Design review of the part built by this model. Coordinates are the model's own, in mm. Face numbers are marked on the shaded views. A direction names the side the tool comes from. Coordinates: 2 decimals unless noted, no trailing zeros. Write each loop counter-clockwise with the first axis right and the second up, starting at its lowest first coordinate (ties: lowest second). Pieces come first, ordered by that corner, then holes. Notation, with made-up numbers: (10.5, 27.25) - (66.5, 27.25) arc R14 ccw to (66.5, 46.25) - close; hole circle Ø5 at (-16.5, -18.5). An arc over 180 degrees is marked (long way). Answer as a JSON object with one key per item and string values.
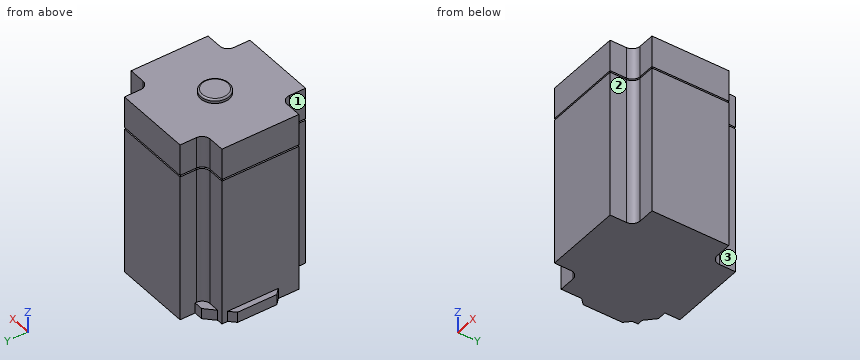
```python
from build123d import *

# Parameters (mm, degrees)
Y_KSEKLIK_EKSTR_ZYON1_DEPTH     = 13
Y_KSEKLIK_EKSTR_ZYON2_DEPTH     = 224
KES_EKSTR_ZYON1_DEPTH           = 1
KES_EKSTR_ZYON1_TAPER           = 45
KES_EKSTR_ZYON1_OTHER_WAY_DEPTH = 1
KES_EKSTR_ZYON1_OTHER_WAY_TAPER = 45
IZIM8_R                         = 17.581787387
Y_KSEKLIK_EKSTR_ZYON3_DEPTH     = 5
RADYUS2_R                       = 2


with BuildPart() as part:
    # Çizim1 → Yükseklik-Ekstrüzyon1 (new body)
    with BuildSketch(Plane.XY):
        Polygon((-58.626768768, 58.968306861), (-84.598484816, 33.394607486), (-84.598484816, -15.059977091), (-58.626768768, -41.031693139), (-10.172184191, -41.031693139), (15.401515184, -15.059977091), (15.401515184, 32.642615461), (-10.924176216, 58.968306861), align=None)
    extrude(amount=Y_KSEKLIK_EKSTR_ZYON1_DEPTH)

    # Çizim2 → Yükseklik-Ekstrüzyon2 (add)
    with BuildSketch(Plane.XY):
        with BuildLine():
            Line((47.5, 57.5), (47.5, 77.5))
            Line((47.5, 77.5), (-47.5, 77.5))
            Line((-47.5, 77.5), (-47.5, 57.5))
            ThreePointArc((-47.5, 57.5), (-50.428932188, 50.428932188), (-57.5, 47.5))
            Line((-57.5, 47.5), (-77.5, 47.5))
            Line((-77.5, 47.5), (-77.5, -47.5))
            Line((-77.5, -47.5), (-57.5, -47.5))
            ThreePointArc((-57.5, -47.5), (-50.428932188, -50.428932188), (-47.5, -57.5))
            Line((-47.5, -57.5), (-47.5, -77.5))
            Line((-47.5, -77.5), (47.5, -77.5))
            Line((47.5, -77.5), (47.5, -57.5))
            ThreePointArc((47.5, -57.5), (50.428932188, -50.428932188), (57.5, -47.5))
            Line((57.5, -47.5), (77.5, -47.5))
            Line((77.5, -47.5), (77.5, 47.5))
            Line((77.5, 47.5), (57.5, 47.5))
            ThreePointArc((57.5, 47.5), (50.428932188, 50.428932188), (47.5, 57.5))
        make_face()
    extrude(amount=Y_KSEKLIK_EKSTR_ZYON2_DEPTH)

    # Çizim7 → Kes-Ekstrüzyon1 (cut)
    with BuildSketch(Plane.XY.offset(184)):
        with BuildLine():
            Line((57.5, -56.5), (86.5, -56.5))
            Line((86.5, -56.5), (86.5, 56.5))
            Line((86.5, 56.5), (57.5, 56.5))
            ThreePointArc((57.5, 56.5), (56.792893219, 56.792893219), (56.5, 57.5))
            Line((56.5, 57.5), (56.5, 86.5))
            Line((56.5, 86.5), (-56.5, 86.5))
            Line((-56.5, 86.5), (-56.5, 57.5))
            ThreePointArc((-56.5, 57.5), (-56.792893219, 56.792893219), (-57.5, 56.5))
            Line((-57.5, 56.5), (-86.5, 56.5))
            Line((-86.5, 56.5), (-86.5, -56.5))
            Line((-86.5, -56.5), (-57.5, -56.5))
            ThreePointArc((-57.5, -56.5), (-56.792893219, -56.792893219), (-56.5, -57.5))
            Line((-56.5, -57.5), (-56.5, -86.5))
            Line((-56.5, -86.5), (56.5, -86.5))
            Line((56.5, -86.5), (56.5, -57.5))
            ThreePointArc((56.5, -57.5), (56.792893219, -56.792893219), (57.5, -56.5))
        make_face()
        with BuildLine():
            Line((-46.5, -76.5), (46.5, -76.5))
            Line((46.5, -76.5), (46.5, -57.5))
            ThreePointArc((46.5, -57.5), (49.721825407, -49.721825407), (57.5, -46.5))
            Line((57.5, -46.5), (76.5, -46.5))
            Line((76.5, -46.5), (76.5, 46.5))
            Line((76.5, 46.5), (57.5, 46.5))
            ThreePointArc((57.5, 46.5), (49.721825407, 49.721825407), (46.5, 57.5))
            Line((46.5, 57.5), (46.5, 76.5))
            Line((46.5, 76.5), (-46.5, 76.5))
            Line((-46.5, 76.5), (-46.5, 57.5))
            ThreePointArc((-46.5, 57.5), (-49.721825407, 49.721825407), (-57.5, 46.5))
            Line((-57.5, 46.5), (-76.5, 46.5))
            Line((-76.5, 46.5), (-76.5, -46.5))
            Line((-76.5, -46.5), (-57.5, -46.5))
            ThreePointArc((-57.5, -46.5), (-49.721825407, -49.721825407), (-46.5, -57.5))
            Line((-46.5, -57.5), (-46.5, -76.5))
        make_face(mode=Mode.SUBTRACT)
    extrude(amount=-KES_EKSTR_ZYON1_DEPTH, taper=KES_EKSTR_ZYON1_TAPER, mode=Mode.SUBTRACT)

    # Çizim7 → Kes-Ekstrüzyon1 other way (cut)
    with BuildSketch(Plane.XY.offset(184)):
        with BuildLine():
            Line((57.5, -56.5), (86.5, -56.5))
            Line((86.5, -56.5), (86.5, 56.5))
            Line((86.5, 56.5), (57.5, 56.5))
            ThreePointArc((57.5, 56.5), (56.792893219, 56.792893219), (56.5, 57.5))
            Line((56.5, 57.5), (56.5, 86.5))
            Line((56.5, 86.5), (-56.5, 86.5))
            Line((-56.5, 86.5), (-56.5, 57.5))
            ThreePointArc((-56.5, 57.5), (-56.792893219, 56.792893219), (-57.5, 56.5))
            Line((-57.5, 56.5), (-86.5, 56.5))
            Line((-86.5, 56.5), (-86.5, -56.5))
            Line((-86.5, -56.5), (-57.5, -56.5))
            ThreePointArc((-57.5, -56.5), (-56.792893219, -56.792893219), (-56.5, -57.5))
            Line((-56.5, -57.5), (-56.5, -86.5))
            Line((-56.5, -86.5), (56.5, -86.5))
            Line((56.5, -86.5), (56.5, -57.5))
            ThreePointArc((56.5, -57.5), (56.792893219, -56.792893219), (57.5, -56.5))
        make_face()
        with BuildLine():
            Line((-46.5, -76.5), (46.5, -76.5))
            Line((46.5, -76.5), (46.5, -57.5))
            ThreePointArc((46.5, -57.5), (49.721825407, -49.721825407), (57.5, -46.5))
            Line((57.5, -46.5), (76.5, -46.5))
            Line((76.5, -46.5), (76.5, 46.5))
            Line((76.5, 46.5), (57.5, 46.5))
            ThreePointArc((57.5, 46.5), (49.721825407, 49.721825407), (46.5, 57.5))
            Line((46.5, 57.5), (46.5, 76.5))
            Line((46.5, 76.5), (-46.5, 76.5))
            Line((-46.5, 76.5), (-46.5, 57.5))
            ThreePointArc((-46.5, 57.5), (-49.721825407, 49.721825407), (-57.5, 46.5))
            Line((-57.5, 46.5), (-76.5, 46.5))
            Line((-76.5, 46.5), (-76.5, -46.5))
            Line((-76.5, -46.5), (-57.5, -46.5))
            ThreePointArc((-57.5, -46.5), (-49.721825407, -49.721825407), (-46.5, -57.5))
            Line((-46.5, -57.5), (-46.5, -76.5))
        make_face(mode=Mode.SUBTRACT)
    extrude(amount=KES_EKSTR_ZYON1_OTHER_WAY_DEPTH, taper=KES_EKSTR_ZYON1_OTHER_WAY_TAPER, mode=Mode.SUBTRACT)

    # Çizim8 → Yükseklik-Ekstrüzyon3 (add)
    with BuildSketch(Plane.XY.offset(224)):
        Circle(IZIM8_R)
    extrude(amount=Y_KSEKLIK_EKSTR_ZYON3_DEPTH)

    # Radyus2
    radyus2_edges = [part.edges().sort_by_distance(p)[0] for p in [
        (-17.581787387, 0, 229),
    ]]
    fillet(radyus2_edges, radius=RADYUS2_R)


solid = part.part
```
(1) To check wall thickness, follow line 1 (Y direction, x = -61, z = 19); line 2 (X direction, y = -11, z = 52.5). State the ranges of each line that lie inside material, in increasing order. Write a range as from..to.
Solved:
{"line 1": "y = -47.5..47.5", "line 2": "x = -77.5..77.5"}
(2) Take a section at A-A, the plane z = 95.5. Write out the cut boundary in (x, y).
Solved:
{"outline": "(-77.5, -47.5) - (-57.5, -47.5) arc R10 cw to (-47.5, -57.5) - (-47.5, -77.5) - (47.5, -77.5) - (47.5, -57.5) arc R10 cw to (57.5, -47.5) - (77.5, -47.5) - (77.5, 47.5) - (57.5, 47.5) arc R10 cw to (47.5, 57.5) - (47.5, 77.5) - (-47.5, 77.5) - (-47.5, 57.5) arc R10 cw to (-57.5, 47.5) - (-77.5, 47.5) - close"}
(3) For pin 1 (6 mm diameter, centred on x = -63, z = 204.5, fed in from -Y); pin 2 (22 mm diameter, centred on x = 67.5, z = 82.5, fed in from +Y); pin 3 (6 mm diameter, centred on y = 65, z = 206.5, fed in from -X), all flat-tipped, find the tip position at first contact; note any pin that passes through.
Solved:
{"pin 1": "stops at y = -47.5", "pin 2": "stops at y = 47.55", "pin 3": "stops at x = -47.5"}
(4) Tool access review of the marked faces 1, 2 and 3: name each direction out of +Z, -Z, +X, -X, +Y, -Y from which nothing blocks a thin tool from reaching the whole face with its end or side.
Solved:
{"face 1": "+Z, -Z, -X, -Y", "face 2": "+Z, -Z, +X, -Y", "face 3": "+Z, -Z, +X, +Y"}
